Work out the finished part from the listing and answer in its coordinate system (mm). A direction names the side the tool comes from. Round coordinates to 2 decimals unless told otherwise and drop trailing zeros. Order: outer loops, then holes, each group sorted by start corner. A loop starts at its lowest first (then second) coordinate and runs counter-clockwise, first axis right, second up. Notation, with made-up numbers: M 16.5,79.5 L 41.5,79.5 A27 cw 41.5,103.5 Z; hole C -17,6.25 d2. An arc over 180 degrees is marked long. Return JSON: item names as keys, results as strings.
from build123d import *

# Parameters (mm, degrees)
F0_W     = 50.8
F0_H     = 19.05
F0_W_2   = 45.72
F0_H_2   = 13.97
F1_DEPTH = 12.7
F2_W     = 50.8
F2_H     = 19.05
F3_DEPTH = 2.54
F5_START = 0.508
F4_W     = 4.572
F4_H     = 2.794
F4_W_2   = 12.7
F4_H_2   = 5.08
F4_H_3   = 3.81
F5_DEPTH = 12.954
F6_R     = 6.34999
F7_W     = 50.8
F7_H     = 19.05
F7_R     = 6.985
F8_DEPTH = 2.54
F9_R     = 2.54
F10_R    = 2.54


# Not quite as in the source:
# - a fillet or chamfer is up to 0.001 mm smaller than in the source, because OpenCascade refuses the exact size


with BuildPart() as f1:
    # F0 (on Top) → F1 (new body)
    with BuildSketch(Plane.XY):
        Rectangle(F0_W, F0_H)
        Rectangle(F0_W_2, F0_H_2, mode=Mode.SUBTRACT)
    extrude(amount=F1_DEPTH)

    # F2 (on face) → F3 (join)
    with BuildSketch(Plane(origin=(0, 0, 0), x_dir=(1, 0, 0), z_dir=(0, 0, -1))):
        Rectangle(F2_W, F2_H)
    extrude(amount=F3_DEPTH)

    # F4 (on face) → F5 (join)
    with BuildSketch(Plane.XZ.offset(-6.985).offset(F5_START)):
        Polygon((-25.4, 0.254), (-25.4, -2.54), (20.828, -2.54), (20.828, 0.254), (-20.828, 0.254), align=None)
        with Locations((23.114, -1.143)):
            Rectangle(F4_W, F4_H)
        with BuildLine():
            Line((-20.828, 0.254), (20.828, 0.254))
            Line((20.828, 0.254), (20.828, 0.508))
            ThreePointArc((20.828, 0.508), (19.7166563034, 0.9891715443), (19.3070802744, 2.1288462099))
            Line((19.3070802744, 2.1288462099), (5.08, 7.62))
            Line((5.08, 7.62), (-5.08, 7.62))
            Line((-5.08, 7.62), (-19.3070802744, 2.1288462099))
            ThreePointArc((-19.3070802744, 2.1288462099), (-19.3047702633, 2.0804475914), (-19.304, 2.032))
            ThreePointArc((-19.304, 2.032), (-19.7503692655, 0.9543692655), (-20.828, 0.508))
            Line((-20.828, 0.508), (-20.828, 0.254))
        make_face()
        with BuildLine():
            ThreePointArc((19.3070802744, 2.1288462099), (19.7166563034, 0.9891715443), (20.828, 0.508))
            Line((20.828, 0.508), (20.828, 2.032))
            Line((20.828, 2.032), (19.558, 2.032))
            Line((19.558, 2.032), (19.3070802744, 2.1288462099))
        make_face()
        with BuildLine():
            Line((20.828, 2.032), (20.828, 0.508))
            ThreePointArc((20.828, 0.508), (21.9056307345, 0.9543692655), (22.352, 2.032))
            ThreePointArc((22.352, 2.032), (21.7251962822, 3.2639151071), (20.3603794867, 3.4824851104))
            Line((20.3603794867, 3.4824851104), (20.828, 3.302))
            Line((20.828, 3.302), (20.828, 2.032))
        make_face()
        with BuildLine():
            ThreePointArc((-20.3603794867, 3.4824851104), (-22.3335091013, 2.2686819509), (-20.828, 0.508))
            Line((-20.828, 0.508), (-20.828, 2.032))
            Line((-20.828, 2.032), (-20.828, 3.302))
            Line((-20.828, 3.302), (-20.3603794867, 3.4824851104))
        make_face()
        with BuildLine():
            Line((-20.828, 2.032), (-20.828, 0.508))
            ThreePointArc((-20.828, 0.508), (-19.7503692655, 0.9543692655), (-19.304, 2.032))
            ThreePointArc((-19.304, 2.032), (-19.3047702633, 2.0804475914), (-19.3070802744, 2.1288462099))
            Line((-19.3070802744, 2.1288462099), (-19.558, 2.032))
            Line((-19.558, 2.032), (-20.828, 2.032))
        make_face()
        with BuildLine():
            Line((19.558, 2.032), (20.828, 2.032))
            Line((20.828, 2.032), (20.828, 3.302))
            Line((20.828, 3.302), (20.3603794867, 3.4824851104))
            ThreePointArc((20.3603794867, 3.4824851104), (19.6252291828, 2.9679051027), (19.3070802744, 2.1288462099))
            Line((19.3070802744, 2.1288462099), (19.558, 2.032))
        make_face()
        with BuildLine():
            Line((5.08, 7.62), (19.3070802744, 2.1288462099))
            ThreePointArc((19.3070802744, 2.1288462099), (19.6252291828, 2.9679051027), (20.3603794867, 3.4824851104))
            Line((20.3603794867, 3.4824851104), (6.35, 8.89))
            Line((6.35, 8.89), (6.35, 7.62))
            Line((6.35, 7.62), (5.08, 7.62))
        make_face()
        with BuildLine():
            Line((-20.828, 3.302), (-20.828, 2.032))
            Line((-20.828, 2.032), (-19.558, 2.032))
            Line((-19.558, 2.032), (-19.3070802744, 2.1288462099))
            ThreePointArc((-19.3070802744, 2.1288462099), (-19.6252291828, 2.9679051027), (-20.3603794867, 3.4824851104))
            Line((-20.3603794867, 3.4824851104), (-20.828, 3.302))
        make_face()
        with BuildLine():
            Line((-6.35, 8.89), (-20.3603794867, 3.4824851104))
            ThreePointArc((-20.3603794867, 3.4824851104), (-19.6252291828, 2.9679051027), (-19.3070802744, 2.1288462099))
            Line((-19.3070802744, 2.1288462099), (-5.08, 7.62))
            Line((-5.08, 7.62), (-6.35, 7.62))
            Line((-6.35, 7.62), (-6.35, 8.89))
        make_face()
        Polygon((-5.08, 7.62), (5.08, 7.62), (6.35, 7.62), (6.35, 8.89), (6.35, 12.7), (-6.35, 12.7), (-6.35, 8.89), (-6.35, 7.62), align=None)
        with Locations((0, 15.24)):
            Rectangle(F4_W_2, F4_H_2)
        with Locations((0, 19.685)):
            Rectangle(F4_W_2, F4_H_3)
    extrude(amount=F5_DEPTH)

    # F6 (radius 6.35 in the source; OpenCascade refuses exactly that, so slightly less here)
    f6_edges = [f1.edges().sort_by_distance(p)[0] for p in [
        (-6.35, -6.477, 15.24),
        (6.35, -6.477, 15.24),
        (6.35, 6.477, 15.24),
        (-6.35, 6.477, 15.24),
    ]]
    fillet(f6_edges, radius=F6_R)

    # F7 (on face) → F8 (join)
    with BuildSketch(Plane.XY.offset(12.7)):
        Rectangle(F7_W, F7_H)
        Circle(F7_R, mode=Mode.SUBTRACT)
    extrude(amount=F8_DEPTH)

    # F9
    f9_edges = [f1.edges().sort_by_distance(p)[0] for p in [
        (-25.4, 9.525, 6.35),
        (-25.4, 0, 15.24),
        (-25.4, -9.525, 6.35),
        (-25.4, 0, -2.54),
        (25.4, 9.525, 6.35),
        (25.4, 0, -2.54),
        (25.4, -9.525, 6.35),
        (25.4, 0, 15.24),
        (0, -9.525, 15.24),
        (0, -9.525, -2.54),
        (0, 9.525, -2.54),
        (0, 9.525, 15.24),
    ]]
    fillet(f9_edges, radius=F9_R)

    # F10
    f10_edges = [f1.edges().sort_by_distance(p)[0] for p in [
        (4.490131, -4.617131, 21.59),
    ]]
    fillet(f10_edges, radius=F10_R)


solid = f1.part
Item 1: Find section A-A (z = 6.25). Determine the outline of the cut face in (x, y) (3 decimals), plus the area to 3 significant figures.
Output:
{"outline": "M -25.4,-6.985 A2.54 ccw -22.86,-9.525 L 22.86,-9.525 A2.54 ccw 25.4,-6.985 L 25.4,6.985 A2.54 ccw 22.86,9.525 L -22.86,9.525 A2.54 ccw -25.4,6.985 Z; M -13.19,-6.477 L 13.19,-6.477 L 13.19,6.477 L -13.19,6.477 Z; hole M -22.86,-6.985 L 22.86,-6.985 L 22.86,6.985 L -22.86,6.985 Z", "area": "665 mm^2"}
Item 2: Find section D-D (z = 12). State how many separate pieces and enclosed holes the cut face has, plus the area to 3 significant figures.
Output:
{"separate pieces": "2", "enclosed holes": "1", "area": "453 mm^2"}
Item 3: Which of the six approach directions +Z, -Z, +X, -X, +Y, -Y give full straight-line access (tool end or side, diameter ignored) to faces 4 (the flat face through (-25.4, 0, 6)), 5 (the flat face through (0, -6.985, 6)), 6 (the cylindrical face through (-0.909, 6.926, 13.952))?
Output:
{"face 4": "+Z, -Z, -X, +Y, -Y", "face 5": "none", "face 6": "+Z"}
Item 4: The mould has two halves that part along Z. Classify faces 1 (the flat face through (12.585, 0.091, 6.484)), 2 (the flat face through (0, 0, 21.59)), 3 (the cylindrical face through (24.636, -8.801, 6.439)): pulls with the +Z half, pulls with the -Z half, needs draft (parallel to the pull), parting line crosses it, or undercut.
Output:
{"face 1": "undercut", "face 2": "pulls with the +Z half", "face 3": "needs draft"}
Item 5: Consider line 1 along Y through (x, z) = (7, 0.5) (3 decimals); line 2 along X through (y, z) = (0, 13.3) (3 decimals); line 3 along X through (y, z) = (0, 14.2) (3 decimals). Determine where each line is inside the solid, lowest interval first. Write a range as [from, to].
Output:
{"line 1": "y = [-9.525, -6.985], [-6.477, 6.477], [6.985, 9.525]", "line 2": "x = [-25.328, -6.985], [-6.35, 6.35], [6.985, 25.328]", "line 3": "x = [-24.91, -6.985], [-6.35, 6.35], [6.985, 24.91]"}
Item 6: Find section B-B (x = -10). Determine the outline of the cut face in (y, z) (3 decimals).
Output:
{"outline": "M -9.525,0 A2.54 ccw -6.985,-2.54 L 6.985,-2.54 A2.54 ccw 9.525,0 L 9.525,12.7 A2.54 ccw 6.985,15.24 L -6.985,15.24 A2.54 ccw -9.525,12.7 Z; hole M -6.985,0 L -6.477,0 L -6.477,7.481 L 6.477,7.481 L 6.477,0 L 6.985,0 L 6.985,12.7 L -6.985,12.7 Z"}
Item 7: Each of these flat-tipped pins is pushed along its axis until it touches: pin 1 (1.6 mm diameter, centred on x = 21.5, y = 2.5, fed in from +Z); pin 2 (10 mm diameter, centred on x = 6.5, z = 15, fed in from +Y) (3 decimals); pin 3 (1 mm diameter, centred on y = -6, z = 17, fed in from +X). Where does it stop, or does it pass through?
Output:
{"pin 1": "stops at z = 15.24", "pin 2": "stops at y = 9.525", "pin 3": "stops at x = 3.38"}
